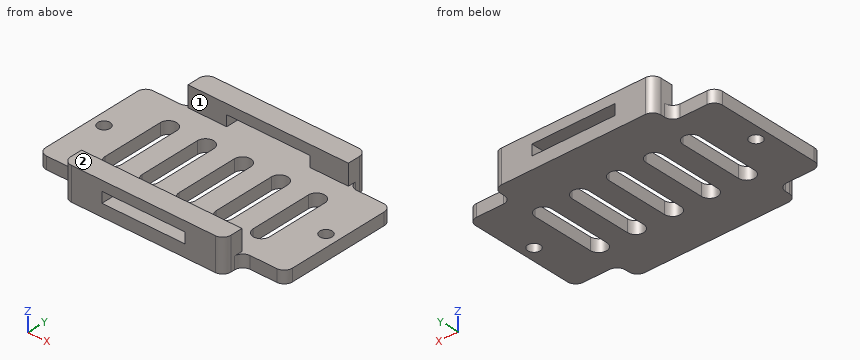
```python
from build123d import *

# Parameters (mm, degrees)
SKETCH_2_W          = 39
SKETCH_2_H          = 5
EXTRUDE_1_DEPTH     = 8
SKETCH_3_W          = 60
SKETCH_3_H          = 3
EXTRUDE_2_DEPTH     = 29
SKETCH_4_W          = 20.2
SKETCH_4_H          = 2.6
CUT_EXTRUDE_1_DEPTH = 47.043457733
SKETCH_5_R          = 1.5
CUT_EXTRUDE_2_DEPTH = 10
FILLET_1_R          = 2
FILLET_2_R          = 2
SKETCH_6_W          = 39
SKETCH_6_H          = 3
EXTRUDE_3_DEPTH     = 5
SKETCH_7_W          = 39
SKETCH_7_H          = 5
EXTRUDE_4_DEPTH     = 5
SKETCH_8_W          = 20.2
SKETCH_8_H          = 2.6
CUT_EXTRUDE_3_DEPTH = 5
FILLET_3_R          = 2
CUT_EXTRUDE_4_DEPTH = 5


with BuildPart() as part:
    # 草图2 → 凸台-拉伸1 (new body)
    with BuildSketch(Plane.XY):
        Rectangle(SKETCH_2_W, SKETCH_2_H)
    extrude(amount=EXTRUDE_1_DEPTH)

    # 草图3 → 凸台-拉伸2 (add)
    with BuildSketch(Plane(origin=(0, 2.5, 0), x_dir=(1, 0, 0), z_dir=(0, 1, 0))):
        with Locations((0, -1.5)):
            Rectangle(SKETCH_3_W, SKETCH_3_H)
    extrude(amount=EXTRUDE_2_DEPTH)

    # 草图4 → 切除-拉伸1 (cut, through all)
    with BuildSketch(Plane.XZ.offset(2.5)):
        with Locations((0, 4.3)):
            Rectangle(SKETCH_4_W, SKETCH_4_H)
    extrude(amount=-CUT_EXTRUDE_1_DEPTH, mode=Mode.SUBTRACT)

    # 草图5 → 切除-拉伸2 (cut)
    with BuildSketch(Plane(origin=(0, 0, 0), x_dir=(-1, 0, 0), z_dir=(0, 0, -1))):
        with Locations((-27, 17)):
            Circle(SKETCH_5_R)
        with Locations((27, 17)):
            Circle(SKETCH_5_R)
    extrude(amount=-CUT_EXTRUDE_2_DEPTH, mode=Mode.SUBTRACT)

    # 圆角1
    fillet_1_edges = [part.edges().sort_by_distance(p)[0] for p in [
        (-30, 2.5, 1.5),
        (30, 2.5, 1.5),
        (-30, 31.5, 1.5),
        (30, 31.5, 1.5),
        (19.5, -2.5, 4),
        (-19.5, -2.5, 4),
    ]]
    fillet(fillet_1_edges, radius=FILLET_1_R)

    # 圆角2
    fillet_2_edges = [part.edges().sort_by_distance(p)[0] for p in [
        (-19.5, 2.5, 1.5),
        (19.5, 2.5, 1.5),
    ]]
    fillet(fillet_2_edges, radius=FILLET_2_R)

    # 草图6 → 凸台-拉伸3 (add)
    with BuildSketch(Plane(origin=(0, 31.5, 0), x_dir=(1, 0, 0), z_dir=(0, 1, 0))):
        with Locations((0, -1.5)):
            Rectangle(SKETCH_6_W, SKETCH_6_H)
    extrude(amount=EXTRUDE_3_DEPTH)

    # 草图7 → 凸台-拉伸4 (add)
    with BuildSketch(Plane.XY.offset(3)):
        with Locations((0, 34)):
            Rectangle(SKETCH_7_W, SKETCH_7_H)
    extrude(amount=EXTRUDE_4_DEPTH)

    # 草图8 → 切除-拉伸3 (cut)
    with BuildSketch(Plane(origin=(0, 36.5, 0), x_dir=(1, 0, 0), z_dir=(0, 1, 0))):
        with Locations((0, -4.3)):
            Rectangle(SKETCH_8_W, SKETCH_8_H)
    extrude(amount=-CUT_EXTRUDE_3_DEPTH, mode=Mode.SUBTRACT)

    # 圆角3
    fillet_3_edges = [part.edges().sort_by_distance(p)[0] for p in [
        (-19.5, 31.5, 1.5),
        (19.5, 31.5, 1.5),
        (-19.5, 36.5, 4),
        (19.5, 36.5, 4),
    ]]
    fillet(fillet_3_edges, radius=FILLET_3_R)

    # 草图9 → 切除-拉伸4 (cut)
    with BuildSketch(Plane(origin=(0, 0, 0), x_dir=(-1, 0, 0), z_dir=(0, 0, -1))):
        with BuildLine():
            Line((2, 24.5), (2, 9.5))
            ThreePointArc((2, 9.5), (0, 7.5), (-2, 9.5))
            Line((-2, 9.5), (-2, 24.5))
            ThreePointArc((-2, 24.5), (0, 26.5), (2, 24.5))
        make_face()
        with BuildLine():
            Line((7, 24.5), (7, 9.5))
            ThreePointArc((7, 9.5), (9, 7.5), (11, 9.5))
            Line((11, 9.5), (11, 24.5))
            ThreePointArc((11, 24.5), (9, 26.5), (7, 24.5))
        make_face()
        with BuildLine():
            Line((16, 24.5), (16, 9.5))
            ThreePointArc((16, 9.5), (18, 7.5), (20, 9.5))
            Line((20, 9.5), (20, 24.5))
            ThreePointArc((20, 24.5), (18, 26.5), (16, 24.5))
        make_face()
        with BuildLine():
            Line((-11, 24.5), (-11, 9.5))
            ThreePointArc((-11, 9.5), (-9, 7.5), (-7, 9.5))
            Line((-7, 9.5), (-7, 24.5))
            ThreePointArc((-7, 24.5), (-9, 26.5), (-11, 24.5))
        make_face()
        with BuildLine():
            Line((-20, 24.5), (-20, 9.5))
            ThreePointArc((-20, 9.5), (-18, 7.5), (-16, 9.5))
            Line((-16, 9.5), (-16, 24.5))
            ThreePointArc((-16, 24.5), (-18, 26.5), (-20, 24.5))
        make_face()
    extrude(amount=-CUT_EXTRUDE_4_DEPTH, mode=Mode.SUBTRACT)


solid = part.part
```
Build history of the part. All positions in model axes, mm. Face numbers are marked on the shaded views. A direction names the side the tool comes from. Give positions to 0.01 mm unless a question says otherwise; leave off trailing zeros. Loops run counter-clockwise (first coordinate to the right, second up) from the corner with the lowest first, then second, coordinate; pieces in that order, holes last. Notation, with made-up numbers: (-25, -13) -> (-10, -13) arc R14 cw to (-10, -8) -> close; hole circle Ø2 at (-38.5, -6.75). An arc over 180 degrees is marked (long way). One line per question, with ' | ' between items. Start each with the question number.
1) Cut at D-D (x = 9). Give the cut face in (y, z), plus the area to 3 significant figures.
2) Cut at A-A (y = 13.5). Give the cut face in (x, z).
3) Probe L1, parallel to X at y = 24.5, z = 2.5; L2, parallel to X at y = 1, z = 4.25; L3, parallel to Y at x = -9, z = 1.5. List the from-to ranges inside material, lowest first.
4) 3-axis set-ups, long thin cutter, end or side, ignore diameter. For the marked faces 1 and 2: which of +Z, -Z, +X, -X, +Y, -Y reach the whole face in a straight line?
5) Cut at C-C (z = 7.25). Give the cut face in (x, y), plus the area to 3 significant figures.
6) Pin check, flat tips, straight feed: pin 1 (3.5 mm diameter, centred on x = 24, z = 1, fed in from +Y); pin 2 (2.5 mm diameter, centred on x = -25, z = 1.5, fed in from -Y); pin 3 (5.5 mm diameter, centred on x = 1, y = 33, fed in from -Z); pin 4 (6 mm diameter, centred on x = 11, y = 22, fed in from +Z). Stop position of each tip, or through.
7) Cut at B-B (x = 3). Give the cut face in (y, z), plus the area to 3 significant figures.
Return value:
1) outline: (-2.5, 0) -> (7.5, 0) -> (7.5, 3) -> (-2.5, 3) -> close; (-2.5, 5.6) -> (2.5, 5.6) -> (2.5, 8) -> (-2.5, 8) -> close; (26.5, 0) -> (36.5, 0) -> (36.5, 3) -> (26.5, 3) -> close; (31.5, 5.6) -> (36.5, 5.6) -> (36.5, 8) -> (31.5, 8) -> close | area: 84.0 mm^2
2) outline: (-30, 0) -> (-20, 0) -> (-20, 3) -> (-30, 3) -> close; (-16, 0) -> (-11, 0) -> (-11, 3) -> (-16, 3) -> close; (-7, 0) -> (-2, 0) -> (-2, 3) -> (-7, 3) -> close; (2, 0) -> (7, 0) -> (7, 3) -> (2, 3) -> close; (11, 0) -> (16, 0) -> (16, 3) -> (11, 3) -> close; (20, 0) -> (30, 0) -> (30, 3) -> (20, 3) -> close
3) L1: -30 to -20, -16 to -11, -7 to -2, 2 to 7, 11 to 16, 20 to 30 | L2: -19.5 to -10.1, 10.1 to 19.5 | L3: -2.5 to 7.5, 26.5 to 36.5
4) face 1: +Z, +X, -X | face 2: +Z, +X, -X, +Y, -Y
5) outline: (-19.5, -0.5) arc R2 ccw to (-17.5, -2.5) -> (17.5, -2.5) arc R2 ccw to (19.5, -0.5) -> (19.5, 2.5) -> (-19.5, 2.5) -> close; (-19.5, 31.5) -> (19.5, 31.5) -> (19.5, 34.5) arc R2 ccw to (17.5, 36.5) -> (-17.5, 36.5) arc R2 ccw to (-19.5, 34.5) -> close | area: 387 mm^2
6) pin 1: y = 31.5 | pin 2: y = 2.5 | pin 3: z = 0 | pin 4: z = 3
7) outline: (-2.5, 0) -> (36.5, 0) -> (36.5, 3) -> (-2.5, 3) -> close; (-2.5, 5.6) -> (2.5, 5.6) -> (2.5, 8) -> (-2.5, 8) -> close; (31.5, 5.6) -> (36.5, 5.6) -> (36.5, 8) -> (31.5, 8) -> close | area: 141 mm^2
